Geometry check sheet. Reference: the model listing, model coordinates, mm. Face numbers are marked on the shaded views. A direction names the side the tool comes from. Give positions to 0.01 mm unless a question says otherwise; leave off trailing zeros. Loops run counter-clockwise (first coordinate to the right, second up) from the corner with the lowest first, then second, coordinate; pieces in that order, holes last. Notation, with made-up numbers: (67, -27) -> (89, -27) arc R9 cw to (89, -20) -> close; hole circle Ø11 at (0, 57.25). An arc over 180 degrees is marked (long way). Write item = value, one per line. Start each with the question number.
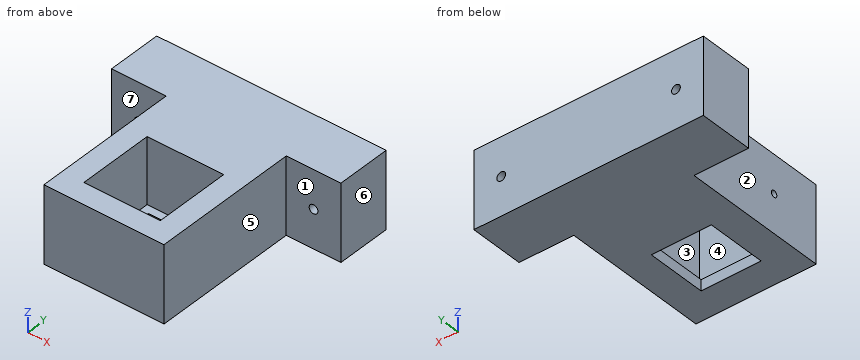
```python
from build123d import *

# Parameters (mm, degrees)
ESQUISSE1_W             = 11
ESQUISSE1_H             = 18.5
BOSS_EXTRU_1_DEPTH      = 7
ESQUISSE2_W             = 7
ESQUISSE2_H             = 7
ENL_V_MAT_EXTRU_1_DEPTH = 6
ESQUISSE4_W             = 5.5
ESQUISSE4_H             = 5.5
ENL_V_MAT_EXTRU_2_DEPTH = 10
ENL_V_MAT_EXTRU_3_REACH = 13
ESQUISSE5_R             = 0.3
ESQUISSE7_W             = 7
ESQUISSE7_H             = 5
BOSS_EXTRU_2_DEPTH      = 5
ESQUISSE8_W             = 7
ESQUISSE8_H             = 5
BOSS_EXTRU_3_DEPTH      = 5
ESQUISSE9_R             = 0.4
ENL_V_MAT_EXTRU_4_DEPTH = 19.5


with BuildPart() as part:
    # Esquisse1 → Boss.-Extru.1 (new body)
    with BuildSketch(Plane.XY):
        with Locations((5.5, 9.25)):
            Rectangle(ESQUISSE1_W, ESQUISSE1_H)
    extrude(amount=BOSS_EXTRU_1_DEPTH)

    # Esquisse2 → Enlèv. mat.-Extru.1 (cut)
    with BuildSketch(Plane.XY.offset(7)):
        with Locations((5.5, 5.5)):
            Rectangle(ESQUISSE2_W, ESQUISSE2_H)
    extrude(amount=-ENL_V_MAT_EXTRU_1_DEPTH, mode=Mode.SUBTRACT)

    # Esquisse4 → Enlèv. mat.-Extru.2 (cut)
    with BuildSketch(Plane.XY.offset(1)):
        with Locations((5.5, 5.5)):
            Rectangle(ESQUISSE4_W, ESQUISSE4_H)
    extrude(amount=-ENL_V_MAT_EXTRU_2_DEPTH, mode=Mode.SUBTRACT)

    # Esquisse5 → Enlèv. mat.-Extru.3 (cut, up to next)
    with BuildSketch(Plane.ZY, mode=Mode.PRIVATE) as enl_v_mat_extru_3_sk1:
        with Locations((3.5, 4.640028524)):
            Circle(ESQUISSE5_R)
    enl_v_mat_extru_3_tool1 = extrude(enl_v_mat_extru_3_sk1.sketch, amount=-ENL_V_MAT_EXTRU_3_REACH, mode=Mode.PRIVATE) & part.part
    add(enl_v_mat_extru_3_tool1.solids().sort_by_distance((0, 4.640029, 3.5))[0], mode=Mode.SUBTRACT)

    # Esquisse7 → Boss.-Extru.2 (add)
    with BuildSketch(Plane(origin=(11, 0, 0), x_dir=(0, 0, -1), z_dir=(1, 0, 0))):
        with Locations((-3.5, 16)):
            Rectangle(ESQUISSE7_W, ESQUISSE7_H)
    extrude(amount=BOSS_EXTRU_2_DEPTH)

    # Esquisse8 → Boss.-Extru.3 (add)
    with BuildSketch(Plane.ZY):
        with Locations((3.5, 16)):
            Rectangle(ESQUISSE8_W, ESQUISSE8_H)
    extrude(amount=BOSS_EXTRU_3_DEPTH)

    # Esquisse9 → Enlèv. mat.-Extru.4 (cut, through all)
    with BuildSketch(Plane(origin=(0, 18.5, 0), x_dir=(1, 0, 0), z_dir=(0, 1, 0))):
        with Locations((-2.5, -3.5)):
            Circle(ESQUISSE9_R)
        with Locations((13.5, -3.5)):
            Circle(ESQUISSE9_R)
    extrude(amount=-ENL_V_MAT_EXTRU_4_DEPTH, mode=Mode.SUBTRACT)


solid = part.part
```
1) Tool access check on the marked faces 4, 5, 6 and 7. Record the directions out of +Z, -Z, +X, -X, +Y, -Y that give a thin tool (end or side, any length) a straight path to the whole face; none if there is none.
2) Section check B-B (x = 13.5). Enter the section's corners in (y, z).
3) Depth check by flat-ended pin: pin 1 Ø0.5 at (y, z) = (4.5, 0.5) entering from +X; pin 2 Ø0.5 at (y, z) = (6, 0.5) entering from -X; pin 3 Ø2.5 at (x, z) = (-3, 4) entering from -Y. Enter the tip coordinate at first touch or a pass-through.
4) Section check A-A (z = 3.5). Enter the section's corners in (x, y).
5) Draft check along X on the marked faces 1, 2 and 3. Enter one of: released by +X, released by -X, zero draft, split by the parting line, or undercut.
6) Section check D-D (z = 0.5). Enter the section's corners in (x, y), plus the area to 3 significant figures.
7) Thickness scan on line 1 (X direction, y = 16.3, z = 3.5); line 2 (Y direction, x = 2.75, z = 1.5); line 3 (X direction, y = 4.5, z = 0.75). Record the ranges inside material, lowest first.
8) Section check C-C (y = 3). Enter the section's corners in (x, z), plus the area to 3 significant figures.
Check result:
q1.face_4 = +Z
q1.face_5 = +Z, -Z, +X, -Y
q1.face_6 = +Z, -Z, +X, +Y, -Y
q1.face_7 = +Z, -Z, -X, -Y
q2.outline = (13.5, 0) -> (18.5, 0) -> (18.5, 3.1) -> (13.5, 3.1) -> close; (13.5, 3.9) -> (18.5, 3.9) -> (18.5, 7) -> (13.5, 7) -> close
q3.pin_1 = 11
q3.pin_2 = 0
q3.pin_3 = 13.5
q4.outline = (-5, 13.5) -> (-2.9, 13.5) -> (-2.9, 18.5) -> (-5, 18.5) -> close; (-2.1, 13.5) -> (0, 13.5) -> (0, 4.94) -> (2, 4.94) -> (2, 9) -> (9, 9) -> (9, 2) -> (2, 2) -> (2, 4.34) -> (0, 4.34) -> (0, 0) -> (11, 0) -> (11, 13.5) -> (13.1, 13.5) -> (13.1, 18.5) -> (-2.1, 18.5) -> close; (13.9, 13.5) -> (16, 13.5) -> (16, 18.5) -> (13.9, 18.5) -> close
q5.face_1 = zero draft
q5.face_2 = released by -X
q5.face_3 = undercut
q6.outline = (-5, 13.5) -> (0, 13.5) -> (0, 0) -> (11, 0) -> (11, 13.5) -> (16, 13.5) -> (16, 18.5) -> (-5, 18.5) -> close; hole (2.75, 2.75) -> (8.25, 2.75) -> (8.25, 8.25) -> (2.75, 8.25) -> close
q6.area = 223 mm2
q7.line_1 = -5 to -2.9, -2.1 to 13.1, 13.9 to 16
q7.line_2 = 0 to 2, 9 to 18.5
q7.line_3 = 0 to 2.75, 8.25 to 11
q8.outline = (0, 0) -> (2.75, 0) -> (2.75, 1) -> (2, 1) -> (2, 7) -> (0, 7) -> close; (8.25, 0) -> (11, 0) -> (11, 7) -> (9, 7) -> (9, 1) -> (8.25, 1) -> close
q8.area = 29.5 mm2
